```python
from build123d import *

# Parameters (mm, degrees)
SKETCH1_W           = 50.8
SKETCH1_H           = 25.4
BOSS_EXTRUDE1_DEPTH = 279.4
SHELL1_T            = -3.175
SKETCH2_R           = 2.38125
CUT_EXTRUDE1_DEPTH  = 282.699627263


with BuildPart() as part:
    # Sketch1 → Boss-Extrude1 (new, symmetric)
    with BuildSketch(Plane(origin=(0, 0, 0), x_dir=(1, 0, 0), z_dir=(0, 1, 0))):
        Rectangle(SKETCH1_W, SKETCH1_H)
    extrude(amount=BOSS_EXTRUDE1_DEPTH, both=True)

    # Shell1
    shell1_openings = [part.faces().sort_by_distance(p)[0] for p in [
        (0, 279.4, 0),
        (0, -279.4, 0),
    ]]
    offset(amount=SHELL1_T, openings=shell1_openings, kind=Kind.INTERSECTION)

    # Sketch2 → Cut-Extrude1 (cut, through all)
    with BuildSketch(Plane(origin=(0, 0, -12.7), x_dir=(-1, 0, 0), z_dir=(0, 0, -1))):
        with Locations((-12.7, -266.7)):
            Circle(SKETCH2_R)
        with Locations((0, -266.7)):
            Circle(SKETCH2_R)
        with Locations((12.7, -266.7)):
            Circle(SKETCH2_R)
        with Locations((-12.7, 266.7)):
            Circle(SKETCH2_R)
        with Locations((-12.7, 241.3)):
            Circle(SKETCH2_R)
        with Locations((12.7, 241.3)):
            Circle(SKETCH2_R)
        with Locations((12.7, 266.7)):
            Circle(SKETCH2_R)
    extrude(amount=-CUT_EXTRUDE1_DEPTH, mode=Mode.SUBTRACT)


solid = part.part
```
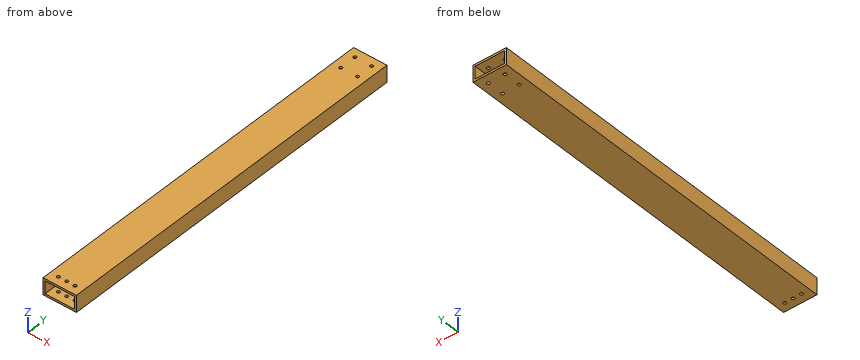
Here's how the part is built. I have some questions about the finished solid (model axes, mm). Round coordinates to 2 decimals unless told otherwise and drop trailing zeros. Order: outer loops, then holes, each group sorted by start corner. A loop starts at its lowest first (then second) coordinate and runs counter-clockwise, first axis right, second up. Notation, with made-up numbers: M 14,-16.5 L 47,-16.5 A24 ccw 47,-4.5 Z; hole C -10.75,88 d5. An arc over 180 degrees is marked long. Answer as CSV lines item,"result".
Item 1: Please list where these lines run through material, in increasing order: L1, parallel to X at y = -266.7, z = 10.4; L2, parallel to X at y = 266.7, z = 10.8; L3, parallel to Y at x = 13, z = -10. Write a range as [from, to].
From the geometry:
L1,"[-25.4, -15.08], [-10.32, -2.38], [2.38, 10.32], [15.08, 25.4]"
L2,"[-25.4, -15.08], [-10.32, 10.32], [15.08, 25.4]"
L3,"[-279.4, -269.06], [-264.34, 238.94], [243.66, 264.34], [269.06, 279.4]"
Item 2: Imagine slicing it at A-A on z = -1. List the corners of the cut face in (x, y) for me (3 decimals).
From the geometry:
outline,"M -25.4,-279.4 L -22.225,-279.4 L -22.225,279.4 L -25.4,279.4 Z; M 22.225,-279.4 L 25.4,-279.4 L 25.4,279.4 L 22.225,279.4 Z"
Item 3: Imagine slicing it at B-B on y = 83.5. List the corners of the cut face in (x, z) for me (3 decimals), and give its area (3 significant figures).
From the geometry:
outline,"M -25.4,-12.7 L 25.4,-12.7 L 25.4,12.7 L -25.4,12.7 Z; hole M -22.225,-9.525 L 22.225,-9.525 L 22.225,9.525 L -22.225,9.525 Z"
area,"444 mm2"
